Source: CAD feature listing. Evaluate the final solid. Frame: model axes, mm. A direction names the side the tool comes from. Round coordinates to 2 decimals unless told otherwise and drop trailing zeros. Use a Markdown table: item, result.
```python
from build123d import *

# Parameters (mm, degrees)
F0_R           = 75
F1_DEPTH       = 12.7
F2_D           = 6.8
F4_D           = 9
F4_CBORE_D     = 14.25
F4_CBORE_DEPTH = 8
F6_D           = 8


# Not quite as in the source:
# - a fillet or chamfer that OpenCascade refuses, or shapes differently, is made with other operations: its cross-section is extruded or revolved along the edge and cut away or added


with BuildPart() as f1:
    # F0 (on Top) → F1 (new body)
    with BuildSketch(Plane.XY):
        Circle(F0_R)
    extrude(amount=F1_DEPTH)

    # F2 (through all)
    with Locations(Plane(origin=(0, 0, 0), x_dir=(1, 0, 0), z_dir=(0, 0, -1))):
        with Locations((-58, -18.8), (0, -61), (58, -18.8), (35.8, 49.3), (-35.8, 49.3)):
            Hole(F2_D / 2)

    # F4 (through all)
    with Locations(Plane.XY.offset(12.7)):
        with Locations((0, 50), (-43.8068557852, 25.8756999398), (42.7956845933, 24.1243000602), (-44.8180269771, -24.1243000602), (-2.0223423839, -50), (41.7845134013, -25.8756999398)):
            CounterBoreHole(F4_D / 2, F4_CBORE_D / 2, F4_CBORE_DEPTH)

    # F5: chamfer of 0.5 on 24 edges, made by hand

    # F5_s1 → F5_t2 (revolve, cut)
    with BuildSketch(Plane.XZ):
        Polygon((75, 12.2), (74.5, 12.7), (75, 12.7), align=None)
    revolve(axis=Axis((0, 0, 12.7), (0, 0, 1)), mode=Mode.SUBTRACT)

    # F5_s3 → F5_t4 (revolve, cut)
    with BuildSketch(Plane.XZ.offset(49.3)):
        Polygon((-31.9, 12.7), (-32.4, 12.2), (-32.4, 12.7), align=None)
    revolve(axis=Axis((-35.8, -49.3, 12.7), (0, 0, -1)), mode=Mode.SUBTRACT)

    # F5_s5 → F5_t6 (revolve, cut)
    with BuildSketch(Plane.XZ.offset(50)):
        Polygon((5.6026576161, 12.7), (5.1026576161, 12.2), (5.1026576161, 12.7), align=None)
    revolve(axis=Axis((-2.0223423839, -50, 12.7), (0, 0, 1)), mode=Mode.SUBTRACT)

    # F5_s7 → F5_t8 (revolve, cut)
    with BuildSketch(Plane.XZ.offset(24.1243000602)):
        Polygon((-37.1930269771, 12.7), (-37.6930269771, 12.2), (-37.6930269771, 12.7), align=None)
    revolve(axis=Axis((-44.8180269771, -24.1243000602, 12.7), (0, 0, 1)), mode=Mode.SUBTRACT)

    # F5_s9 → F5_t10 (revolve, cut)
    with BuildSketch(Plane.XZ.offset(49.3)):
        Polygon((39.7, 12.7), (39.2, 12.2), (39.2, 12.7), align=None)
    revolve(axis=Axis((35.8, -49.3, 12.7), (0, 0, -1)), mode=Mode.SUBTRACT)

    # F5_s11 → F5_t12 (revolve, cut)
    with BuildSketch(Plane.XZ.offset(25.8756999398)):
        Polygon((49.4095134013, 12.7), (48.9095134013, 12.2), (48.9095134013, 12.7), align=None)
    revolve(axis=Axis((41.7845134013, -25.8756999398, 12.7), (0, 0, 1)), mode=Mode.SUBTRACT)

    # F5_s13 → F5_t14 (revolve, cut)
    with BuildSketch(Plane.XZ.offset(-18.8)):
        Polygon((-54.1, 12.7), (-54.6, 12.2), (-54.6, 12.7), align=None)
    revolve(axis=Axis((-58, 18.8, 12.7), (0, 0, -1)), mode=Mode.SUBTRACT)

    # F5_s15 → F5_t16 (revolve, cut)
    with BuildSketch(Plane.XZ.offset(-25.8756999398)):
        Polygon((-36.1818557852, 12.7), (-36.6818557852, 12.2), (-36.6818557852, 12.7), align=None)
    revolve(axis=Axis((-43.8068557852, 25.8756999398, 12.7), (0, 0, 1)), mode=Mode.SUBTRACT)

    # F5_s17 → F5_t18 (revolve, cut)
    with BuildSketch(Plane.XZ.offset(-18.8)):
        Polygon((61.9, 12.7), (61.4, 12.2), (61.4, 12.7), align=None)
    revolve(axis=Axis((58, 18.8, 12.7), (0, 0, -1)), mode=Mode.SUBTRACT)

    # F5_s19 → F5_t20 (revolve, cut)
    with BuildSketch(Plane.XZ.offset(-24.1243000602)):
        Polygon((50.4206845933, 12.7), (49.9206845933, 12.2), (49.9206845933, 12.7), align=None)
    revolve(axis=Axis((42.7956845933, 24.1243000602, 12.7), (0, 0, 1)), mode=Mode.SUBTRACT)

    # F5_s21 → F5_t22 (revolve, cut)
    with BuildSketch(Plane.XZ.offset(-50)):
        Polygon((7.625, 12.7), (7.125, 12.2), (7.125, 12.7), align=None)
    revolve(axis=Axis((0, 50, 12.7), (0, 0, 1)), mode=Mode.SUBTRACT)

    # F5_s23 → F5_t24 (revolve, cut)
    with BuildSketch(Plane.XZ.offset(-61)):
        Polygon((3.9, 12.7), (3.4, 12.2), (3.4, 12.7), align=None)
    revolve(axis=Axis((0, 61, 12.7), (0, 0, -1)), mode=Mode.SUBTRACT)

    # F5_s25 → F5_t26 (revolve, cut)
    with BuildSketch(Plane.XZ):
        Polygon((75, 0.5), (74.5, 0), (75, 0), align=None)
    revolve(axis=Axis((0, 0, 0), (0, 0, 1)), mode=Mode.SUBTRACT)

    # F5_s27 → F5_t28 (revolve, cut)
    with BuildSketch(Plane.XZ.offset(49.3)):
        Polygon((-31.9, 0), (-32.4, 0.5), (-32.4, 0), align=None)
    revolve(axis=Axis((-35.8, -49.3, 0), (0, 0, -1)), mode=Mode.SUBTRACT)

    # F5_s29 → F5_t30 (revolve, cut)
    with BuildSketch(Plane.XZ.offset(50)):
        Polygon((2.9776576161, 0), (2.4776576161, 0.5), (2.4776576161, 0), align=None)
    revolve(axis=Axis((-2.0223423839, -50, 0), (0, 0, 1)), mode=Mode.SUBTRACT)

    # F5_s31 → F5_t32 (revolve, cut)
    with BuildSketch(Plane.XZ.offset(24.1243000602)):
        Polygon((-39.8180269771, 0), (-40.3180269771, 0.5), (-40.3180269771, 0), align=None)
    revolve(axis=Axis((-44.8180269771, -24.1243000602, 0), (0, 0, 1)), mode=Mode.SUBTRACT)

    # F5_s33 → F5_t34 (revolve, cut)
    with BuildSketch(Plane.XZ.offset(49.3)):
        Polygon((39.7, 0), (39.2, 0.5), (39.2, 0), align=None)
    revolve(axis=Axis((35.8, -49.3, 0), (0, 0, -1)), mode=Mode.SUBTRACT)

    # F5_s35 → F5_t36 (revolve, cut)
    with BuildSketch(Plane.XZ.offset(25.8756999398)):
        Polygon((46.7845134013, 0), (46.2845134013, 0.5), (46.2845134013, 0), align=None)
    revolve(axis=Axis((41.7845134013, -25.8756999398, 0), (0, 0, 1)), mode=Mode.SUBTRACT)

    # F5_s37 → F5_t38 (revolve, cut)
    with BuildSketch(Plane.XZ.offset(-18.8)):
        Polygon((-54.1, 0), (-54.6, 0.5), (-54.6, 0), align=None)
    revolve(axis=Axis((-58, 18.8, 0), (0, 0, -1)), mode=Mode.SUBTRACT)

    # F5_s39 → F5_t40 (revolve, cut)
    with BuildSketch(Plane.XZ.offset(-25.8756999398)):
        Polygon((-38.8068557852, 0), (-39.3068557852, 0.5), (-39.3068557852, 0), align=None)
    revolve(axis=Axis((-43.8068557852, 25.8756999398, 0), (0, 0, 1)), mode=Mode.SUBTRACT)

    # F5_s41 → F5_t42 (revolve, cut)
    with BuildSketch(Plane.XZ.offset(-18.8)):
        Polygon((61.9, 0), (61.4, 0.5), (61.4, 0), align=None)
    revolve(axis=Axis((58, 18.8, 0), (0, 0, -1)), mode=Mode.SUBTRACT)

    # F5_s43 → F5_t44 (revolve, cut)
    with BuildSketch(Plane.XZ.offset(-24.1243000602)):
        Polygon((47.7956845933, 0), (47.2956845933, 0.5), (47.2956845933, 0), align=None)
    revolve(axis=Axis((42.7956845933, 24.1243000602, 0), (0, 0, 1)), mode=Mode.SUBTRACT)

    # F5_s45 → F5_t46 (revolve, cut)
    with BuildSketch(Plane.XZ.offset(-50)):
        Polygon((5, 0), (4.5, 0.5), (4.5, 0), align=None)
    revolve(axis=Axis((0, 50, 0), (0, 0, 1)), mode=Mode.SUBTRACT)

    # F5_s47 → F5_t48 (revolve, cut)
    with BuildSketch(Plane.XZ.offset(-61)):
        Polygon((3.9, 0), (3.4, 0.5), (3.4, 0), align=None)
    revolve(axis=Axis((0, 61, 0), (0, 0, -1)), mode=Mode.SUBTRACT)

    # F6 (through all)
    with Locations(Plane.XY.offset(12.7)):
        with Locations((-51.0111711919, 0), (48.9888288081, 0)):
            Hole(F6_D / 2)


solid = f1.part
```
Q1. Section A-A on z = 9. Give the number of separate pieces and of enclosed holes in the cut face, plus the area to 3 significant figures.
Results are:
| item | result |
|---|---|
| separate pieces | 1 |
| enclosed holes | 13 |
| area | 16,400 mm^2 |
Q2. Reachability of faces 1 (the cylindrical face through (-37.4, -46.3, 6.4)), 2 (the flat face through (3, -50, 4.7)) from +Z, -Z, +X, -X, +Y, -Y: full face, straight path, thin tool, end or side. Return the list, or none.
Results are:
| item | result |
|---|---|
| face 1 | +Z, -Z |
| face 2 | +Z |
Q3. Mould query, pull axis X, two halves, no side actions, for faces 3 (the cylindrical face through (-50.925, 26.189, 8.502)), 4 (the conical face through (-1.574, 42.912, 12.335)), 5 (the flat face through (-1, 1, 12.7)). Classes: +X half, -X half, draft (parallel to the pull), parting line (faces both ways), or undercut.
Results are:
| item | result |
|---|---|
| face 3 | undercut |
| face 4 | undercut |
| face 5 | draft |
Q4. First-contact query: pin 1 Ø8 at (x, y) = (41.78, -25.88) entering from +Z; pin 2 Ø18.5 at (x, y) = (-2.02, -50) entering from -Z; pin 3 Ø1 at (x, z) = (13, 4) entering from +Y; pin 4 Ø1.5 at (x, z) = (-26, 4.5) entering from +Y. Flat tips, straight axial feed; report the tip coordinate or a pass-through.
Results are:
| item | result |
|---|---|
| pin 1 | through |
| pin 2 | z = 0 |
| pin 3 | y = 73.95 |
| pin 4 | y = 70.62 |
Q5. Line query: L1, parallel to Y at x = 44, z = 6.5; L2, parallel to Y at x = -2, z = 6.5; L3, parallel to X at y = -23.5, z = 1.25. Output: solid intervals per line, ascending.
Results are:
| item | result |
|---|---|
| L1 | -60.74 to -32.65, -19.1 to 17.1, 31.15 to 60.74 |
| L2 | -74.97 to -57.12, -42.88 to 43.16, 56.84 to 58.25, 63.75 to 74.97 |
| L3 | -71.22 to -49.27, -40.36 to 37.96, 45.61 to 71.22 |
